```python
from build123d import *

# Parameters (mm, degrees)
SKETCH1_W           = 6.35
SKETCH1_H           = 6.35
BOSS_EXTRUDE1_DEPTH = 3.81
SKETCH2_W           = 1.78977558
SKETCH2_H           = 1.018153585
BOSS_EXTRUDE2_DEPTH = 0.254
SKETCH3_R           = 0.508
BOSS_EXTRUDE3_DEPTH = 0.254
FILLET1_R           = 0.254
SKETCH4_R           = 1.363047184
BOSS_EXTRUDE4_DEPTH = 0.508
SKETCH5_R           = 2.2733
BOSS_EXTRUDE5_DEPTH = 6.096


with BuildPart() as part:
    # Sketch1 → Boss-Extrude1 (new body)
    with BuildSketch(Plane(origin=(0, 0, 0), x_dir=(1, 0, 0), z_dir=(0, 1, 0))):
        Rectangle(SKETCH1_W, SKETCH1_H)
    extrude(amount=BOSS_EXTRUDE1_DEPTH)

    # Sketch2 → Boss-Extrude2 (add)
    with BuildSketch(Plane.XZ):
        with Locations((-4.06988779, -2.386523208)):
            Rectangle(SKETCH2_W, SKETCH2_H)
        with Locations((-4.06988779, 2.386523208)):
            Rectangle(SKETCH2_W, SKETCH2_H)
        with Locations((4.06988779, 2.386523208)):
            Rectangle(SKETCH2_W, SKETCH2_H)
        with Locations((4.06988779, -2.386523208)):
            Rectangle(SKETCH2_W, SKETCH2_H)
    extrude(amount=-BOSS_EXTRUDE2_DEPTH)

    # Sketch3 → Boss-Extrude3 (add)
    with BuildSketch(Plane(origin=(0, 3.81, 0), x_dir=(-1, 0, 0), z_dir=(0, 1, 0))):
        with Locations(Location((2.526830598, -2.521609873, 0), (0, 0, 270))):
            Circle(SKETCH3_R)
        with Locations(Location((-2.526830598, -2.521609873, 0), (0, 0, 270))):
            Circle(SKETCH3_R)
        with Locations(Location((-2.526830598, 2.521609873, 0), (0, 0, 270))):
            Circle(SKETCH3_R)
        with Locations(Location((2.526830598, 2.521609873, 0), (0, 0, 270))):
            Circle(SKETCH3_R)
    extrude(amount=BOSS_EXTRUDE3_DEPTH)

    # Fillet1
    fillet1_edges = [part.edges().sort_by_distance(p)[0] for p in [
        (-2.526830598, 4.064, -2.013609873),
        (2.526830598, 4.064, -2.013609873),
        (2.526830598, 4.064, 3.029609873),
        (-2.526830598, 4.064, 3.029609873),
    ]]
    fillet(fillet1_edges, radius=FILLET1_R - 0.0001)  # a hair under: the kernel refuses the full size

    # Sketch4 → Boss-Extrude4 (add)
    with BuildSketch(Plane(origin=(0, 3.81, 0), x_dir=(1, 0, 0), z_dir=(0, 1, 0))):
        with Locations(Location((0, 0, 0), (0, 0, 90))):
            Circle(SKETCH4_R)
    extrude(amount=BOSS_EXTRUDE4_DEPTH)

    # Sketch5 → Boss-Extrude5 (add)
    with BuildSketch(Plane(origin=(0, 4.318, 0), x_dir=(-1, 0, 0), z_dir=(0, 1, 0))):
        with Locations(Location((0, 0, 0), (0, 0, 270))):
            Circle(SKETCH5_R)
    extrude(amount=BOSS_EXTRUDE5_DEPTH)


solid = part.part
```
Can you work these out from the model? Positions are in its coordinate system, mm. A direction names the side the tool comes from. Coordinates: 2 decimals unless noted, no trailing zeros. Loops run counter-clockwise (first coordinate to the right, second up) from the corner with the lowest first, then second, coordinate; pieces in that order, holes last. Notation, with made-up numbers: (24, 4.25) - (40, 4.25) arc R21 cw to (40, 15.25) - close; hole circle Ø4 at (65, 85). An arc over 180 degrees is marked (long way). Answer as CSV lines item,"result". Start each with the question number.
1) Suppose I cut it at A-A (x = -4.5). Please give me the cut outline in (y, z), plus the area to 3 significant figures.
2) Suppose I cut it at C-C (x = 0). Please give me the cut outline in (y, z) (3 decimals).
3) Which directions (+Z, -Z, +X, -X, +Y, -Y) give clear straight access to the entire face, cutting with the end or side of a thin tool? Please do faces 1 (the cylindrical face through (-0.921, 4.06, 1.005)), 2 (the flat face through (-4.1, 0.254, -2.4)), 3 (the flat face through (0, 10.414, 0)), 4 (the flat face through (4.1, 0.254, 2.4)).
4) Suppose I cut it at D-D (y = 8.75). Please give me the cut outline in (x, z), plus the area to 3 significant figures.
5) Suppose I cut it at B-B (z = 0). Please give me the cut outline in (x, y) (3 decimals), plus the area to 3 significant figures.
6) For pin 1 (1.9 mm diameter, centred on y = 1, z = 0, fed in from -X) (3 decimals); pin 2 (2 mm diameter, centred on y = 1.5, z = -2.5, fed in from +X) (3 decimals); pin 3 (1 mm diameter, centred on y = 8.5, z = -1.5, fed in from +X); pin 4 (1.5 mm diameter, centred on x = 3.5, y = 8.5, fed in from +Z), each with a flat end and sliding along its axis, tell me the tip position at first contact or that it passes through.
7) Thinking about a two-plate mould opening in X: for faces 5 (the cylindrical face through (-2.254, 7.323, 0.296)), 6 (the flat face through (1.4, 3.81, 0.7)), 7 (the flat face through (-4.1, 0.254, 2.4)), which applies, pulls with the +X half, pulls with the -X half, needs draft (parallel to the pull), parting line crosses it, or undercut?
8) I need wall thicknesses on line 1 (Y direction, x = -0.25, z = 2); line 2 (Y direction, x = 3, z = 1.5); line 3 (Y direction, x = -2.75, z = 2.5). Which ranges of each line are inside material? Lowest first, please. Write a range as from..to.
Check result:
1,outline,"(0, -2.9) - (0.25, -2.9) - (0.25, -1.88) - (0, -1.88) - close; (0, 1.88) - (0.25, 1.88) - (0.25, 2.9) - (0, 2.9) - close"
1,area,"0.517 mm²"
2,outline,"(0, -3.175) - (3.81, -3.175) - (3.81, -1.363) - (4.318, -1.363) - (4.318, -2.273) - (10.414, -2.273) - (10.414, 2.273) - (4.318, 2.273) - (4.318, 1.363) - (3.81, 1.363) - (3.81, 3.175) - (0, 3.175) - close"
3,face 1,"none"
3,face 2,"+Z, -Z, -X, +Y"
3,face 3,"+Z, -Z, +X, -X, +Y"
3,face 4,"+Z, -Z, +X, +Y"
4,outline,"circle Ø4.55 at (0, 0)"
4,area,"16.2 mm²"
5,outline,"(-3.175, 0) - (3.175, 0) - (3.175, 3.81) - (1.363, 3.81) - (1.363, 4.318) - (2.273, 4.318) - (2.273, 10.414) - (-2.273, 10.414) - (-2.273, 4.318) - (-1.363, 4.318) - (-1.363, 3.81) - (-3.175, 3.81) - close"
5,area,"53.3 mm²"
6,pin 1,"stops at x = -3.175"
6,pin 2,"stops at x = 3.175"
6,pin 3,"stops at x = 2.04"
6,pin 4,"passes through"
7,face 5,"parting line crosses it"
7,face 6,"undercut"
7,face 7,"needs draft"
8,line 1,"y = 0..3.81, 4.32..10.41"
8,line 2,"y = 0..3.81"
8,line 3,"y = 0..4.06"
